Verification items for this drawing (mm, ordinates from the low corner). Round coordinates to 2 decimals unless told otherwise and drop trailing zeros. Loops run counter-clockwise (first coordinate to the right, second up) from the corner with the lowest first, then second, coordinate; pieces in that order, holes last. Notation, with made-up numbers: M 65,9 L 107,9 A20 cw 107,29 Z; hole C 64.25,-12 d10. An arc over 180 degrees is marked long. One line per item, written item: value.
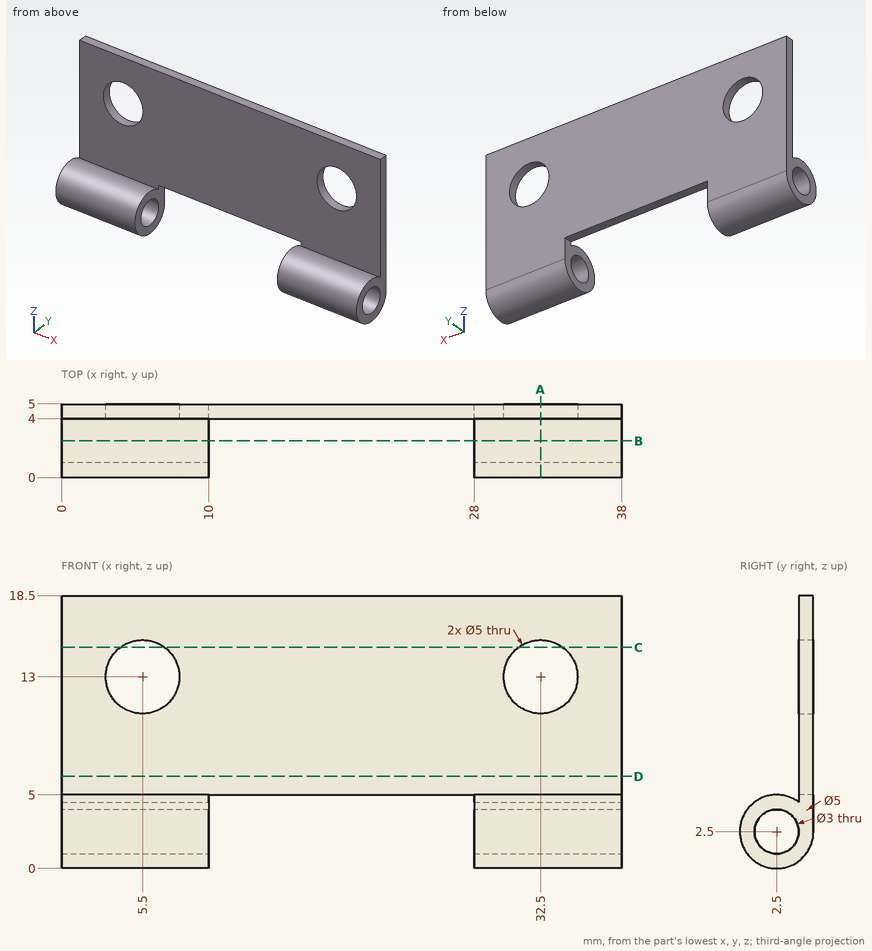
(1) Sectioned sample at B-B on y = 2.5. Enter the section's corners in (x, z).
Completed:
outline: M 0,0 L 10,0 L 10,1 L 0,1 Z; M 0,4 L 10,4 L 10,5 L 0,5 Z; M 28,0 L 38,0 L 38,1 L 28,1 Z; M 28,4 L 38,4 L 38,5 L 28,5 Z
(2) Depth check by flat-ended pin: pin 1 Ø6.5 at (x, z) = (32.5, 13) entering from -Y; pin 2 Ø0.5 at (x, y) = (23.5, 4.5) entering from -Z. Enter the tip coordinate at first touch or a pass-through.
Completed:
pin 1: stops at y = 4
pin 2: stops at z = 5
(3) Sectioned sample at A-A on x = 32.5. Enter the section's corners in (y, z).
Completed:
outline: M 4,4.5 A2.5 ccw long 5,2.5 L 5,10.5 L 4,10.5 Z; M 4,15.5 L 5,15.5 L 5,18.5 L 4,18.5 Z; hole C 2.5,2.5 d3
(4) Thickness scan on L1, parallel to X at y = 4.2, z = 13; L2, parallel to Z at x = 32.25, y = 2.5; L3, parallel to X at y = 4.6, z = 11.25. Record the ranges inside material, lowest first. Write a range as from..to.
Completed:
L1: x = 0..3, 8..30, 35..38
L2: z = 0..1, 4..5
L3: x = 0..3.71, 7.29..30.71, 34.29..38
(5) Sectioned sample at D-D on z = 6.25. Enter the section's corners in (x, y).
Completed:
outline: M 0,4 L 38,4 L 38,5 L 0,5 Z
(6) Sectioned sample at C-C on z = 15. Enter the section's corners in (x, y).
Completed:
outline: M 0,4 L 4,4 L 4,5 L 0,5 Z; M 7,4 L 31,4 L 31,5 L 7,5 Z; M 34,4 L 38,4 L 38,5 L 34,5 Z
